Can you work these out from the model? Positions are in its coordinate system, mm. A direction names the side the tool comes from. Coordinates: 2 decimals unless noted, no trailing zeros. Order: outer loops, then holes, each group sorted by start corner. A loop starts at its lowest first (then second) coordinate and runs counter-clockwise, first axis right, second up.
```python
from build123d import *

# Parameters (mm, degrees)
F0_W      = 35.4
F0_H      = 15.7
F1_DEPTH  = 42.7
F3_DEPTH  = 3.7
F5_DEPTH  = 6
F6_R      = 11.7
F7_DEPTH  = 35
F8_R      = 14.25
F9_DEPTH  = 25
F10_R     = 1.25
F11_DEPTH = 4.5
F12_R     = 1.75
F13_DEPTH = 25
F14_R     = 3
F14_R_2   = 1.75
F15_DEPTH = 7.85


with BuildPart() as f1:
    # F0 (on Top) → F1 (new body)
    with BuildSketch(Plane.XY):
        with Locations((17.7, 7.85)):
            Rectangle(F0_W, F0_H)
    extrude(amount=F1_DEPTH)

    # F2 (on face) → F3 (cut)
    with BuildSketch(Plane.XY.offset(42.7)):
        with BuildLine():
            ThreePointArc((9.7, 15.7), (17.7, 7.7), (25.7, 15.7))
            Line((25.7, 15.7), (9.7, 15.7))
        make_face()
    extrude(amount=-F3_DEPTH, mode=Mode.SUBTRACT)

    # F4 (on face) → F5 (cut)
    with BuildSketch(Plane.XY.offset(39)):
        with BuildLine():
            ThreePointArc((11.45, 15.7), (17.7, 9.45), (23.95, 15.7))
            Line((23.95, 15.7), (11.45, 15.7))
        make_face()
    extrude(amount=-F5_DEPTH, mode=Mode.SUBTRACT)

    # F6 (on face) → F7 (cut)
    with BuildSketch(Plane.XY.offset(33)):
        with Locations((17.7, 15.7)):
            Circle(F6_R)
        with BuildLine():
            Line((11.45, 15.7), (23.95, 15.7))
            ThreePointArc((23.95, 15.7), (17.7, 9.45), (11.45, 15.7))
        make_face(mode=Mode.SUBTRACT)
        with BuildLine():
            ThreePointArc((11.45, 15.7), (17.7, 9.45), (23.95, 15.7))
            Line((23.95, 15.7), (11.45, 15.7))
        make_face()
    extrude(amount=-F7_DEPTH, mode=Mode.SUBTRACT)

    # F8 (on face) → F9 (cut)
    with BuildSketch(Plane.XZ):
        with Locations((17.7, 17.7)):
            Circle(F8_R)
    extrude(amount=-F9_DEPTH, mode=Mode.SUBTRACT)

    # F10 (on face) → F11 (cut)
    with BuildSketch(Plane.XZ):
        with Locations((5.2, 5.5)):
            Circle(F10_R)
        with Locations((5.2, 29.5)):
            Circle(F10_R)
        with Locations((30.2, 29.5)):
            Circle(F10_R)
        with Locations((30.2, 5.5)):
            Circle(F10_R)
    extrude(amount=-F11_DEPTH, mode=Mode.SUBTRACT)

    # F12 (on face) → F13 (cut)
    with BuildSketch(Plane(origin=(0, 15.7, 0), x_dir=(-1, 0, 0), z_dir=(0, 1, 0))):
        with Locations((-4.6, 37.7)):
            Circle(F12_R)
        with Locations((-30.8, 37.7)):
            Circle(F12_R)
    extrude(amount=-F13_DEPTH, mode=Mode.SUBTRACT)

    # F14 (on face) → F15 (cut)
    with BuildSketch(Plane.XZ):
        with Locations((4.6, 37.7)):
            Circle(F14_R)
        with Locations((4.6, 37.7)):
            Circle(F14_R_2, mode=Mode.SUBTRACT)
        with Locations((30.8, 37.7)):
            Circle(F14_R)
        with Locations((30.8, 37.7)):
            Circle(F14_R_2, mode=Mode.SUBTRACT)
    extrude(amount=-F15_DEPTH, mode=Mode.SUBTRACT)


solid = f1.part
```
1. Thinking about a two-plate mould opening in Z: for faces 1 (the flat face through (0, 8, 21)), 2 (the cylindrical face through (28.59, 3.87, 39.73)), 3 (the flat face through (17, 3, 0)), which applies, pulls with the +Z half, pulls with the -Z half, needs draft (parallel to the pull), parting line crosses it, or undercut?
Completed:
face 1: needs draft
face 2: undercut
face 3: pulls with the -Z half
2. Please list where these lines run through material, in increasing order: probe 1 along X at (y, z) = (8.5, 17.7); probe 2 along Z at (x, y) = (6, 8.75); probe 3 along X at (y, z) = (13.75, 38).
Completed:
probe 1: x = 0 to 3.45, 31.95 to 35.4
probe 2: z = 0 to 9.57, 25.83 to 36.65, 38.75 to 42.7
probe 3: x = 0 to 2.88, 6.32 to 11.76, 23.64 to 29.08, 32.52 to 35.4
3. Imagine slicing it at D-D on z = 38.5. Please give me the cut outline in (x, y).
Completed:
outline: (0, 0) - (1.71, 0) - (1.71, 7.85) - (3.04, 7.85) - (3.04, 15.7) - (0, 15.7) - close; (6.16, 7.85) - (7.49, 7.85) - (7.49, 0) - (27.91, 0) - (27.91, 7.85) - (29.24, 7.85) - (29.24, 15.7) - (23.95, 15.7) arc R6.25 cw to (11.45, 15.7) - (6.16, 15.7) - close; (32.36, 7.85) - (33.69, 7.85) - (33.69, 0) - (35.4, 0) - (35.4, 15.7) - (32.36, 15.7) - close
4. Imagine slicing it at C-C on z = 17. Please give me the cut outline in (x, y), then the cut area to 3 significant figures.
Completed:
outline: (0, 0) - (3.47, 0) - (3.47, 15.7) - (0, 15.7) - close; (31.93, 0) - (35.4, 0) - (35.4, 15.7) - (31.93, 15.7) - close
area: 109 mm2
5. I'm going to push flat-ended pins straight in: pin 1 (1.5 mm diameter, centred on x = 30.2, z = 29.5, fed in from -Y); pin 2 (4 mm diameter, centred on x = 21.5, z = 30.5, fed in from +Y); pin 3 (5 mm diameter, centred on x = 4.6, z = 37.7, fed in from -Y). Where does each tip first touch, or does it pass through?
Completed:
pin 1: stops at y = 4.5
pin 2: stops at y = 5.53
pin 3: stops at y = 7.85
6. Imagine slicing it at A-A on x = 17.7. Please give me the cut outline in (y, z), then the cut area to 3 significant figures.
Completed:
outline: (0, 0) - (4, 0) - (4, 3.45) - (0, 3.45) - close; (0, 31.95) - (4, 31.95) - (4, 33) - (9.45, 33) - (9.45, 39) - (7.7, 39) - (7.7, 42.7) - (0, 42.7) - close
area: 103 mm2
7. On a 3-axis mill with a long thin cutter (end or side, diameter ignored), from which of +Z, -Z, +X, -X, +Y, -Y can I reach the whole of each face in a straight line? I mean faces 4 (the cylindrical face through (4.93, 2.22, 4.28)), 5 (the cylindrical face through (17.524, 7.702, 40.876)), 6 (the cylindrical face through (17.443, 4.003, 2.724)), 7 (the cylindrical face through (17.56, 9.45, 36.04)), 8 (the cylindrical face through (32.19, 11.83, 36.64)). Say none if no direction works.
Completed:
face 4: -Y
face 5: +Z, +Y
face 6: -Z, +Y
face 7: +Z, -Z, +Y
face 8: +Y, -Y
8. Imagine slicing it at B-B on y = 13.25. Please give me the cut outline in (x, z).
Completed:
outline: (0, 0) - (6.26, 0) - (6.26, 9.2) arc R14.25 cw to (6.26, 26.2) - (6.26, 33) - (11.95, 33) - (11.95, 39) - (10.08, 39) - (10.08, 42.7) - (0, 42.7) - close; (23.45, 33) - (29.14, 33) - (29.14, 26.2) arc R14.25 cw to (29.14, 9.2) - (29.14, 0) - (35.4, 0) - (35.4, 42.7) - (25.32, 42.7) - (25.32, 39) - (23.45, 39) - close; hole circle Ø3.5 at (4.6, 37.7); hole circle Ø3.5 at (30.8, 37.7)
